from build123d import *

# Parameters (mm, degrees)
F0_W     = 76.9356526434
F0_H     = 79.423185253
F1_DEPTH = 25


# Not quite as in the source:
# - ends of sketch curves that miss each other by under 0.0002 mm in the source are joined


with BuildPart() as f1:
    # F0 (on Front) → F1 (new body)
    with BuildSketch(Plane.XZ):
        Rectangle(F0_W, F0_H)
        with BuildLine():
            Line((11.4050824274, -9.8430258844), (11.4050824274, 29.2284450168))
            ThreePointArc((11.4050824274, 29.2284450168), (16.4050836887, 34.228446278), (21.4050849499, 29.2284450168))
            Line((21.4050849499, 29.2284450168), (21.4050824274, -9.8430258844))
            ThreePointArc((21.4050824274, -9.8430258844), (15.1356789363, -24.9787048207), (0, -31.2481083118))
            Line((0, -31.2481083118), (-19.8113770242, -31.2481083118))
            ThreePointArc((-19.8113770242, -31.2481083118), (-24.8113770242, -26.2481083118), (-19.8113770242, -21.2481083118))
            Line((-19.8113770242, -21.2481083118), (0, -21.2481083118))
            ThreePointArc((0, -21.2481083118), (8.0646111244, -17.9076370088), (11.4050824274, -9.8430258844))
        make_face(mode=Mode.SUBTRACT)
    extrude(amount=F1_DEPTH)


solid = f1.part
Geometry: final body of the model. Coordinates: model frame, mm. A direction names the side the tool comes from. Give positions to 0.01 mm unless a question says otherwise; leave off trailing zeros. Order: outer loops, then holes, each group sorted by start corner. A loop starts at its lowest first (then second) coordinate and runs counter-clockwise, first axis right, second up. Notation, with made-up numbers: (40, -30.5) -> (68, -30.5) arc R12 ccw to (68, -21.5) -> close; hole circle Ø3 at (-23, 13). An arc over 180 degrees is marked (long way). Put each result on its own line as item: value.
Q1. Section C-C, the plane z = -3.5. Return loops of the section in (x, y), then the cut area to 3 significant figures.
Here are the results:
outline: (-38.47, -25) -> (11.41, -25) -> (11.41, 0) -> (-38.47, 0) -> close; (21.41, -25) -> (38.47, -25) -> (38.47, 0) -> (21.41, 0) -> close
area: 1,670 mm^2
Q2. Section A-A, the plane x = -17. Return loops of the section in (y, z).
Here are the results:
outline: (-25, -39.71) -> (0, -39.71) -> (0, -31.25) -> (-25, -31.25) -> close; (-25, -21.25) -> (0, -21.25) -> (0, 39.71) -> (-25, 39.71) -> close
Q3. Material intervals for L1, parallel to X at y = -15.25, z = 24; L2, parallel to Z at x = -20, y = -17.75; L3, parallel to Z at x = -3.5, y = -7.25, sorted ascending.
Here are the results:
L1: x = -38.47 to 11.41, 21.41 to 38.47
L2: z = -39.71 to -31.24, -21.25 to 39.71
L3: z = -39.71 to -31.25, -21.25 to 39.71
Q4. Reachability of faces 1 (the face through (-1, -25, 1)), 2 (the face through (11.405, -12, 9)) from +Z, -Z, +X, -X, +Y, -Y: full face, straight path, thin tool, end or side. Return the list, or none.
Here are the results:
face 1: +Z, -Z, +X, -X, -Y
face 2: +Y, -Y
Q5. Section B-B, the plane y = -14.5. Return loops of the section in (x, z).
Here are the results:
outline: (-38.47, -39.71) -> (38.47, -39.71) -> (38.47, 39.71) -> (-38.47, 39.71) -> close; hole (-19.81, -31.25) -> (0, -31.25) arc R21.41 ccw to (21.41, -9.84) -> (21.41, 29.23) arc R5 ccw to (11.41, 29.23) -> (11.41, -9.84) arc R11.41 cw to (0, -21.25) -> (-19.81, -21.25) arc R5 ccw to start
Q6. Pin query (flat end, axial travel): pin 1 (4 mm diameter, centred on x = -15, z = -28.5, fed in from +Y). Return the tip coordinate at first contact, or that it passes through.
Here are the results:
pin 1: passes through
Q7. Draft query along Z for faces 3 (the face through (16.295, -12.325, 34.227)), 4 (the face through (-10, -12, -21.248)), 5 (the face through (38.468, -12, -1)), 6 (the face through (-1, -12, -39.712)). Return one class per face: released by +Z, released by -Z, zero draft, split by the parting line, or undercut.
Here are the results:
face 3: undercut
face 4: undercut
face 5: zero draft
face 6: released by -Z
